Input: part model. Units: mm. Frame: model coordinates. Round coordinates to 2 decimals unless told otherwise and drop trailing zeros. Loops run counter-clockwise (first coordinate to the right, second up) from the corner with the lowest first, then second, coordinate; pieces in that order, holes last.
1) First-contact query: pin 1 (6.5 mm diameter, centred on x = -120.42, y = -59.43, fed in from -Z); pin 2 (3 mm diameter, centred on y = -318.5, z = 2, fed in from -X); pin 3 (1.8 mm diameter, centred on y = -295.5, z = 4, fed in from -X). Flat tips, straight axial feed; report the tip coordinate or a pass-through.
2) Section A-A, the plane z = 4.45. Return loops of the section in (x, y).
3) Ray query, line 1 along Y through (x, z) = (-28, 1.1); line 2 along Y through (x, z) = (-118, 0.95); line 3 along Y through (x, z) = (-108.5, 5.4). Return the intervals inside material, ascending.
from build123d import *

# Parameters (mm, degrees)
BOSS_EXTRUDE1_DEPTH = 6
SKETCH2_R           = 2.75
CUT_EXTRUDE1_DEPTH  = 10


with BuildPart() as part:
    # Sketch1 → Boss-Extrude1 (new body)
    with BuildSketch(Plane.XY):
        Polygon((-82.419020993, -326.855738356), (-82.419020993, -305.855738356), (-109.419020993, -305.855738356), (-109.419020993, -281.0269235), (-130.419020993, -281.0269235), (-130.419020993, 162.175301007), (-109.419020993, 162.175301007), (-109.419020993, 209.144261644), (-20.419020993, 209.144261644), (-20.419020993, -326.855738356), align=None)
    extrude(amount=BOSS_EXTRUDE1_DEPTH)

    # Sketch2 → Cut-Extrude1 (cut)
    with BuildSketch(Plane.XY.offset(6)):
        with Locations((-120.419020993, -59.425811246)):
            Circle(SKETCH2_R)
        with Locations((-30.419020993, -59.425811246)):
            Circle(SKETCH2_R)
        with Locations((-30.419020993, 174.944215352)):
            Circle(SKETCH2_R)
        with Locations((-30.419020993, -284.937648356)):
            Circle(SKETCH2_R)
        with Locations((-120.419020993, -238.562803654)):
            Circle(SKETCH2_R)
        with Locations((-120.419020993, 132.455525643)):
            Circle(SKETCH2_R)
    extrude(amount=-CUT_EXTRUDE1_DEPTH, mode=Mode.SUBTRACT)


solid = part.part
Final values:
1. pin 1: stops at z = 0
1. pin 2: stops at x = -82.42
1. pin 3: stops at x = -109.42
2. outline: (-130.42, -281.03) - (-109.42, -281.03) - (-109.42, -305.86) - (-82.42, -305.86) - (-82.42, -326.86) - (-20.42, -326.86) - (-20.42, 209.14) - (-109.42, 209.14) - (-109.42, 162.18) - (-130.42, 162.18) - close; hole circle Ø5.5 at (-120.42, -238.56); hole circle Ø5.5 at (-120.42, -59.43); hole circle Ø5.5 at (-120.42, 132.46); hole circle Ø5.5 at (-30.42, -284.94); hole circle Ø5.5 at (-30.42, -59.43); hole circle Ø5.5 at (-30.42, 174.94)
3. line 1: y = -326.86 to -286.25, -283.63 to -60.73, -58.12 to 173.64, 176.25 to 209.14
3. line 2: y = -281.03 to -239.87, -237.25 to -60.73, -58.12 to 131.15, 133.76 to 162.18
3. line 3: y = -305.86 to 209.14
